from build123d import *

# Parameters (mm, degrees)
BOSS_EXTRUDE1_DEPTH = 1
SKETCH2_W           = 50
SKETCH2_H           = 50
BOSS_EXTRUDE2_DEPTH = 1
CUT_EXTRUDE1_DEPTH  = 1


with BuildPart() as part:
    # Sketch1 → Boss-Extrude1 (new body)
    with BuildSketch(Plane(origin=(0, 0, 0), x_dir=(1, 0, 0), z_dir=(0, 1, 0))):
        Polygon((-200, 25), (-174.5, 0), (0, 0), (0, 50), (-200, 50), align=None)
        with BuildLine():
            ThreePointArc((-174.5, 21), (-178.5, 25), (-174.5, 29))
            Line((-174.5, 29), (-144.7, 29))
            ThreePointArc((-144.7, 29), (-140.7, 25), (-144.7, 21))
            Line((-144.7, 21), (-174.5, 21))
        make_face(mode=Mode.SUBTRACT)
        with BuildLine():
            ThreePointArc((-75, 21), (-79, 25), (-75, 29))
            Line((-75, 29), (-15.08, 29))
            ThreePointArc((-15.08, 29), (-11.08, 25), (-15.08, 21))
            Line((-15.08, 21), (-75, 21))
        make_face(mode=Mode.SUBTRACT)
    extrude(amount=BOSS_EXTRUDE1_DEPTH)

    # Sketch2 → Boss-Extrude2 (add)
    with BuildSketch(Plane(origin=(0, 0, 0), x_dir=(0, 0, -1), z_dir=(1, 0, 0))):
        with Locations((25, -24)):
            Rectangle(SKETCH2_W, SKETCH2_H)
    extrude(amount=-BOSS_EXTRUDE2_DEPTH)

    # Sketch3 → Cut-Extrude1 (cut)
    with BuildSketch(Plane(origin=(0, 0, 0), x_dir=(0, 0, -1), z_dir=(1, 0, 0))):
        with BuildLine():
            Line((29, -8.58942274), (29, -32.915209985))
            ThreePointArc((29, -32.915209985), (25, -36.915209985), (21, -32.915209985))
            Line((21, -32.915209985), (21, -8.58942274))
            ThreePointArc((21, -8.58942274), (25, -4.58942274), (29, -8.58942274))
        make_face()
    extrude(amount=-CUT_EXTRUDE1_DEPTH, mode=Mode.SUBTRACT)


solid = part.part
Design review of the part built by this model. Coordinates are the model's own, in mm. A direction names the side the tool comes from. Give positions to 0.01 mm unless a question says otherwise; leave off trailing zeros. Order: outer loops, then holes, each group sorted by start corner. A loop starts at its lowest first (then second) coordinate and runs counter-clockwise, first axis right, second up. Notation, with made-up numbers: (21.25, -31) - (65.25, -31) arc R14 ccw to (65.25, -21) - close; hole circle Ø11 at (45, 44). An arc over 180 degrees is marked (long way). Write item = value, one per line. Start each with the question number.
Q1. We need section C-C on z = -38.5. State the section outline as (x, y) points, plus the area to 3 significant figures.
Q2. We need section A-A on y = -26.5. State the section outline as (x, z) points.
Q3. We need section B-B on x = -19. State the section outline as (y, z) points, plus the area to 3 significant figures.
Q4. Tool access review of faces 5 (the face through (-101, 1, -25)), 6 (the face through (-11.08, 0.49, -25.09)), 7 (the face through (-1, -24, -19)), 8 (the face through (-0.49, -4.59, -24.91)): name each direction out of +Z, -Z, +X, -X, +Y, -Y from which nothing blocks a thin tool from reaching the whole face with its end or side.
Q5. To check wall thickness, follow L1, parallel to Y at x = -143, z = -18; L2, parallel to X at y = -26.5, z = -10. State the ranges of each line that lie inside material, in increasing order. Write a range as from..to.
Q6. We need section D-D on x = -85. State the section outline as (y, z) points.
Q7. Clearance check with flat-ended pins moving along their axes: pin 1 Ø3 at (y, z) = (-36.5, -8) entering from -X; pin 2 Ø2 at (x, z) = (-98.5, -38.5) entering from -Y. State where each tip first meets the part, or that it passes through.
Q8. Mouldability with a two-part tool opening along Z and no side actions: class faces 1 (the face through (-0.493, -36.914, -25.088)), 2 (the face through (-187.428, 0.493, -12.675)), 3 (the face through (-140.7, 0.5, -25.1)), 4 (the face through (-102, 0, -25)) as released by +Z, released by -Z, zero draft, split by the parting line, or undercut.
Working result:
q1.outline = (-200, 0) - (-1, 0) - (-1, -49) - (0, -49) - (0, 1) - (-200, 1) - close
q1.area = 249 mm²
q2.outline = (-1, -50) - (0, -50) - (0, -29) - (-1, -29) - close; (-1, -21) - (0, -21) - (0, 0) - (-1, 0) - close
q3.outline = (0, -50) - (1, -50) - (1, -29) - (0, -29) - close; (0, -21) - (1, -21) - (1, 0) - (0, 0) - close
q3.area = 42.0 mm²
q4.face_5 = +Z, -Z, +X, -X, +Y
q4.face_6 = +Y, -Y
q4.face_7 = +Z, -Z, -X, -Y
q4.face_8 = +X, -X
q5.L1 = 0..1
q5.L2 = -1..0
q6.outline = (0, -50) - (1, -50) - (1, 0) - (0, 0) - close
q7.pin_1 = -1
q7.pin_2 = 0
q8.face_1 = undercut
q8.face_2 = released by +Z
q8.face_3 = undercut
q8.face_4 = zero draft
